Check sheet for the modelled part. Datum: model origin and axes. Units: mm. A direction names the side the tool comes from. Round coordinates to 2 decimals unless told otherwise and drop trailing zeros. Write each loop counter-clockwise with the first axis right and the second up, starting at its lowest first coordinate (ties: lowest second). Pieces come first, ordered by that corner, then holes. Notation, with made-up numbers: M -15.5,88 L 20.5,88 A28 ccw 20.5,127 Z; hole C -0.5,-8 d4. An arc over 180 degrees is marked long. Put each result on its own line as item: value.
```python
from build123d import *

# Parameters (mm, degrees)
F0_R     = 12.75
F0_R_2   = 1.35
F0_R_3   = 1.75
F1_DEPTH = 6.5
F2_R     = 4.35
F3_DEPTH = 4


with BuildPart() as f1:
    # F0 (on Top) → F1 (new body)
    with BuildSketch(Plane.XY):
        Circle(F0_R)
        with Locations((0, -9.7)):
            Circle(F0_R_2, mode=Mode.SUBTRACT)
        Circle(F0_R_3, mode=Mode.SUBTRACT)
        with Locations((0, 9.7)):
            Circle(F0_R_2, mode=Mode.SUBTRACT)
    extrude(amount=F1_DEPTH)

    # F2 (on face) → F3 (cut)
    with BuildSketch(Plane.XY.offset(6.5)):
        Circle(F2_R)
    extrude(amount=-F3_DEPTH, mode=Mode.SUBTRACT)


solid = f1.part
```
1. Access from +Z, -Z, +X, -X, +Y, -Y to the whole of each face (thin tool, end or side, straight path). Record for faces 1 (the cylindrical face through (-0.943, -4.247, 4.528)), 2 (the cylindrical face through (-0.176, 11.039, 3.204)).
Computed values:
face 1: +Z
face 2: +Z, -Z
2. Scan lines: probe 1 along Y at (x, z) = (0, 3.9); probe 2 along Y at (x, z) = (0, 1.8); probe 3 along Y at (x, z) = (-3.75, 4). Record each from-to range of solid material in increasing order.
Computed values:
probe 1: y = -12.75 to -11.05, -8.35 to -4.35, 4.35 to 8.35, 11.05 to 12.75
probe 2: y = -12.75 to -11.05, -8.35 to -1.75, 1.75 to 8.35, 11.05 to 12.75
probe 3: y = -12.19 to -2.2, 2.2 to 12.19
3. Release check for a two-part mould opening along Y. For faces 3 (the cylindrical face through (-2.764, -12.447, 3.204)), 4 (the flat face through (0, -3, 0)), 5 (the flat face through (0, -2, 2.5)) record: +Y half, -Y half, draft (parallel to the pull), parting line (faces both ways), or undercut.
Computed values:
face 3: parting line
face 4: draft
face 5: undercut
4. Depth check by flat-ended pin: pin 1 Ø4 at (x, y) = (0, 0) entering from +Z; pin 2 Ø12 at (x, y) = (3.5, 3.5) entering from -Z; pin 3 Ø1.5 at (y, z) = (8.5, 4) entering from +X. Enter the tip coordinate at first touch or a pass-through.
Computed values:
pin 1: stops at z = 2.5
pin 2: stops at z = 0
pin 3: stops at x = 10.12
5. Cross-section at A-A (x = 0). Enter the section's corners in (y, z), then the cut area to 3 significant figures.
Computed values:
outline: M -12.75,0 L -11.05,0 L -11.05,6.5 L -12.75,6.5 Z; M -8.35,0 L -1.75,0 L -1.75,2.5 L -4.35,2.5 L -4.35,6.5 L -8.35,6.5 Z; M 1.75,0 L 8.35,0 L 8.35,6.5 L 4.35,6.5 L 4.35,2.5 L 1.75,2.5 Z; M 11.05,0 L 12.75,0 L 12.75,6.5 L 11.05,6.5 Z
area: 87.1 mm2
6. Cross-section at C-C (z = 4.5). Enter the section's corners in (x, y).
Computed values:
outline: C 0,0 d25.5; hole C 0,0 d8.7; hole C 0,-9.7 d2.7; hole C 0,9.7 d2.7
7. Cross-section at D-D (x = -2.75). Enter the section's corners in (y, z).
Computed values:
outline: M -12.45,0 L 12.45,0 L 12.45,6.5 L 3.37,6.5 L 3.37,2.5 L -3.37,2.5 L -3.37,6.5 L -12.45,6.5 Z
8. Cross-section at B-B (y = 0). Enter the section's corners in (x, z).
Computed values:
outline: M -12.75,0 L -1.75,0 L -1.75,2.5 L -4.35,2.5 L -4.35,6.5 L -12.75,6.5 Z; M 1.75,0 L 12.75,0 L 12.75,6.5 L 4.35,6.5 L 4.35,2.5 L 1.75,2.5 Z
